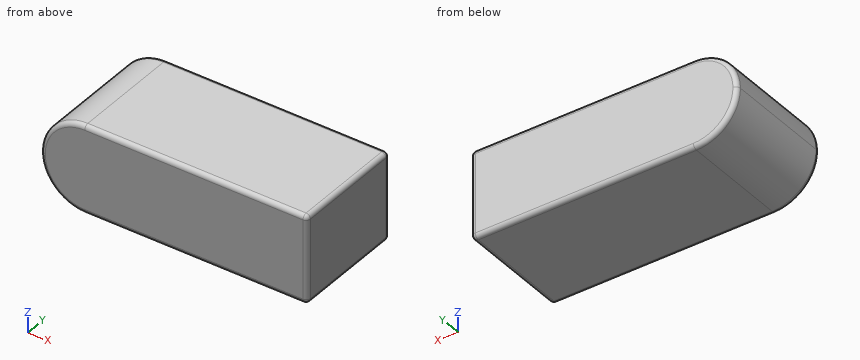
from build123d import *

# Parameters (mm, degrees)
SKETCH1_W           = 77.1525
SKETCH1_H           = 33.2359
BOSS_EXTRUDE1_DEPTH = 25.4
CUT_EXTRUDE1_DEPTH  = 57.902654708
FILLET1_R           = 1.27


with BuildPart() as part:
    # Sketch1 → Boss-Extrude1 (new body)
    with BuildSketch(Plane.XY):
        Rectangle(SKETCH1_W, SKETCH1_H)
    extrude(amount=BOSS_EXTRUDE1_DEPTH)

    # Sketch2 → Cut-Extrude1 (cut, through all)
    with BuildSketch(Plane(origin=(0, 16.61795, 0), x_dir=(1, 0, 0), z_dir=(0, 1, 0))):
        with BuildLine():
            Line((-25.87625, 0), (-51.27625, 0))
            Line((-51.27625, 0), (-51.27625, -25.4))
            Line((-51.27625, -25.4), (-25.87625, -25.4))
            ThreePointArc((-25.87625, -25.4), (-34.856506121, -21.680256121), (-38.57625, -12.7))
            ThreePointArc((-38.57625, -12.7), (-34.856506121, -3.719743879), (-25.87625, 0))
        make_face()
    extrude(amount=-CUT_EXTRUDE1_DEPTH, mode=Mode.SUBTRACT)

    # Fillet1
    fillet1_edges = [part.edges().sort_by_distance(p)[0] for p in [
        (6.35, -16.61795, 0),
        (6.35, -16.61795, 25.4),
        (-38.57625, -16.61795, 12.7),
        (-38.57625, 16.61795, 12.7),
        (38.57625, 0, 25.4),
        (6.35, 16.61795, 0),
        (38.57625, 0, 0),
        (38.57625, -16.61795, 12.7),
        (38.57625, 16.61795, 12.7),
        (6.35, 16.61795, 25.4),
    ]]
    fillet(fillet1_edges, radius=FILLET1_R)


solid = part.part
Source: CAD feature listing. Evaluate the final solid. Frame: model axes, mm. Round coordinates to 2 decimals unless told otherwise and drop trailing zeros. Loops run counter-clockwise (first coordinate to the right, second up) from the corner with the lowest first, then second, coordinate; pieces in that order, holes last. Notation, with made-up numbers: (56.25, 69.25) - (97.25, 69.25) arc R23 cw to (97.25, 98.25) - close; hole circle Ø8 at (-6, -16). An arc over 180 degrees is marked (long way). Write item = value, one per line. Start each with the question number.
Item 1: Section query A-A on y = 2.5. Output: boundary loops of the cut face in (x, z).
Item 2: First-contact query: pin 1 Ø4 at (y, z) = (1.5, 7.5) entering from -X. Flat tip, straight axial feed; report the tip coordinate or a pass-through.
Item 3: Material intervals for line 1 (X direction, y = -1.5, z = 13); line 2 (X direction, y = -10, z = 1); line 3 (Z direction, x = -28, y = 1), sorted ascending.
Results list:
q1.outline = (-25.88, 0) - (37.31, 0) arc R1.27 ccw to (38.58, 1.27) - (38.58, 24.13) arc R1.27 ccw to (37.31, 25.4) - (-25.88, 25.4) arc R12.7 ccw to start
q2.pin_1 = -38.17
q3.line_1 = -38.57 to 38.58
q3.line_2 = -30.82 to 38.55
q3.line_3 = 0.18 to 25.22
